Verification items for the finished model (mm, model axes). A direction names the side the tool comes from. Round coordinates to 2 decimals unless told otherwise and drop trailing zeros. Order: outer loops, then holes, each group sorted by start corner. A loop starts at its lowest first (then second) coordinate and runs counter-clockwise, first axis right, second up.
```python
from build123d import *

# Parameters (mm, degrees)
EXTRUDE_1_DEPTH     = 9
CUT_EXTRUDE_2_DEPTH = 4
SKETCH_7_W          = 6
SKETCH_7_H          = 6
CUT_EXTRUDE_4_DEPTH = 7
SKETCH_10_W         = 6
SKETCH_10_H         = 6
CUT_EXTRUDE_6_DEPTH = 7
SHELL_1_T           = -1.5
SKETCH_5_R          = 1.1
CUT_EXTRUDE_3_DEPTH = 4
CUT_EXTRUDE_START   = -9
SKETCH_6_R          = 1
CUT_EXTRUDE_5_DEPTH = 7.5
FILLET_1_R          = 2
CUT_EXTRUDE_7_REACH = 4
SKETCH_12_R         = 1


with BuildPart() as part:
    # 草图1 → 凸台-拉伸1 (new body)
    with BuildSketch(Plane.XY):
        Polygon((70.444808084, 16.058078986), (70.444808084, -68.941921014), (155.445322416, -68.941921014), (155.444808084, 16.058078986), align=None)
    extrude(amount=EXTRUDE_1_DEPTH)

    # 草图4 → 支架切除-拉伸2 (cut)
    with BuildSketch(Plane.XY.offset(9)):
        Polygon((112.94506525, 16.058078986), (70.444808084, 16.058078986), (70.444808084, -68.941921014), (112.94506525, -68.941921014), (112.94506525, -64.941921014), (74.444808084, -64.941921014), (74.444808084, 12.058078986), (112.94506525, 12.058078986), align=None)
    extrude(amount=-CUT_EXTRUDE_2_DEPTH, mode=Mode.SUBTRACT)

    # 草图7 → 顶螺丝切除-拉伸4 (cut)
    with BuildSketch(Plane.XY.offset(9)):
        with Locations((152.445322416, 13.058078986)):
            Rectangle(SKETCH_7_W, SKETCH_7_H)
        with Locations((152.445322416, -65.941921014)):
            Rectangle(SKETCH_7_W, SKETCH_7_H)
    extrude(amount=-CUT_EXTRUDE_4_DEPTH, mode=Mode.SUBTRACT)

    # 草图10 → 底螺丝切除-拉伸6 (cut)
    with BuildSketch(Plane.XY.offset(9)):
        with Locations((119.944808084, 13.058078986)):
            Rectangle(SKETCH_10_W, SKETCH_10_H)
        with Locations((101.094808084, -65.941921014)):
            Rectangle(SKETCH_10_W, SKETCH_10_H)
    extrude(amount=-CUT_EXTRUDE_6_DEPTH, mode=Mode.SUBTRACT)

    # 抽壳1
    shell_1_openings = [part.faces().sort_by_distance(p)[0] for p in [
        (112.94506525, -26.441921014, 0),
    ]]
    offset(amount=SHELL_1_T, openings=shell_1_openings, kind=Kind.INTERSECTION)

    # 草图5 → 切除-拉伸3 (cut)
    with BuildSketch(Plane(origin=(0, 12.058078986, 0), x_dir=(1, 0, 0), z_dir=(0, 1, 0))):
        with Locations((110.94506525, -7)):
            Circle(SKETCH_5_R)
    cut_extrude_3 = extrude(amount=-CUT_EXTRUDE_3_DEPTH, mode=Mode.SUBTRACT)

    # 镜向1: 切除-拉伸3 across plane
    add(cut_extrude_3.mirror(Plane.ZX.offset(-26.441921014)), mode=Mode.SUBTRACT)

    # 草图6 → 顶螺丝切除-拉伸5 (cut)
    with BuildSketch(Plane.XY.offset(9).offset(CUT_EXTRUDE_START)):
        with Locations((152.344808084, 12.958078986)):
            Circle(SKETCH_6_R)
        with Locations((152.344808084, -65.841921014)):
            Circle(SKETCH_6_R)
    extrude(amount=CUT_EXTRUDE_5_DEPTH, mode=Mode.SUBTRACT)

    # 圆角1
    fillet_1_edges = [part.edges().sort_by_distance(p)[0] for p in [
        (131.195193833, -68.941921014, 9),
        (70.444808084, 16.058078986, 2.5),
        (70.444808084, -68.941921014, 2.5),
        (70.444808084, -26.441921014, 5),
        (74.444808084, -26.441921014, 9),
        (155.44506525, -26.441921014, 9),
        (136.19506525, 16.058078986, 9),
        (155.444808084, 16.058078986, 1),
        (155.445322416, -68.941921014, 1),
        (114.944936667, 16.058078986, 9),
    ]]
    fillet(fillet_1_edges, radius=FILLET_1_R)

    # 草图12 → 底螺丝切除-拉伸7 (cut, up to next)
    with BuildSketch(Plane.XY.offset(2), mode=Mode.PRIVATE) as cut_extrude_7_sk1:
        with Locations((119.944808084, 12.958078986)):
            Circle(SKETCH_12_R)
    cut_extrude_7_tool1 = extrude(cut_extrude_7_sk1.sketch, amount=-CUT_EXTRUDE_7_REACH, mode=Mode.PRIVATE) & part.part
    add(cut_extrude_7_tool1.solids().sort_by_distance((119.944808, 12.958079, 2))[0], mode=Mode.SUBTRACT)
    # 草图12 → 底螺丝切除-拉伸7 (cut, up to next)
    with BuildSketch(Plane.XY.offset(2), mode=Mode.PRIVATE) as cut_extrude_7_sk2:
        with Locations((101.094808084, -65.841921014)):
            Circle(SKETCH_12_R)
    cut_extrude_7_tool2 = extrude(cut_extrude_7_sk2.sketch, amount=-CUT_EXTRUDE_7_REACH, mode=Mode.PRIVATE) & part.part
    add(cut_extrude_7_tool2.solids().sort_by_distance((101.094808, -65.841921, 2))[0], mode=Mode.SUBTRACT)


solid = part.part
```
1) Sectioned sample at A-A on x = 107. Record the cut outline in (y, z).
2) Scan lines: probe 1 along X at (y, z) = (-63.15, 7); probe 2 along X at (y, z) = (-29, 5.75); probe 3 along Y at (x, z) = (91, 3.75). Record each from-to range of solid material in increasing order.
3) Tool access check on faces 5 (the flat face through (86, -64.942, 7)), 6 (the flat face through (116.945, 13, 6)), 7 (the flat face through (152, -62.942, 6)), 8 (the flat face through (151, -61.442, 4)). Record the directions out of +Z, -Z, +X, -X, +Y, -Y that give a thin tool (end or side, any length) a straight path to the whole face; none if there is none.
4) Go/stop test with flat-tipped pins: pin 1 Ø2 at (x, z) = (87.5, 7.5) entering from -Y; pin 2 Ø1.8 at (y, z) = (13.5, 7) entering from +X; pin 3 Ø2 at (x, y) = (110.5, -68) entering from +Z. Record where each tip stops, or that it passes through.
5) Draft check along Z on faces 1 (the cylindrical face through (110.707, 10.531, 8.074)), 2 (the cylindrical face through (153.3, -65.54, 1.24)), 3 (the cylindrical face through (71.015, -27.037, 4.399)), 4 (the flat face through (94, 15, 0)). Enter one of: released by +Z, released by -Z, zero draft, split by the parting line, or undercut.
Returned:
1. outline: (-68.94, 0) - (-67.44, 0) - (-67.44, 3.5) - (-63.44, 3.5) - (-63.44, 7.5) - (10.56, 7.5) - (10.56, 3.5) - (14.56, 3.5) - (14.56, 0) - (16.06, 0) - (16.06, 5) - (12.06, 5) - (12.06, 9) - (-64.94, 9) - (-64.94, 5) - (-68.94, 5) - close
2. probe 1: x = 74.44 to 75.94, 96.59 to 98.09, 104.09 to 105.59, 147.95 to 149.45
2. probe 2: x = 74.44 to 75.94, 153.95 to 155.45
2. probe 3: y = -68.94 to -63.44, 10.56 to 16.06
3. face 5: +Z, -X, -Y
3. face 6: +Z, +Y
3. face 7: +Z, +X, -Y
3. face 8: -Z
4. pin 1: stops at y = -64.94
4. pin 2: stops at x = 149.45
4. pin 3: stops at z = 5
5. face 1: undercut
5. face 2: zero draft
5. face 3: released by +Z
5. face 4: released by -Z
